The listing builds one solid part. Answer for the finished solid, in the listing's coordinates (mm). A direction names the side the tool comes from. Coordinates: 2 decimals unless noted, no trailing zeros. Loops run counter-clockwise (first coordinate to the right, second up) from the corner with the lowest first, then second, coordinate; pieces in that order, holes last. Notation, with made-up numbers: M 51.5,-19 L 93.5,-19 A23 ccw 93.5,4 Z; hole C -22,78.5 d7. An arc over 180 degrees is marked long. Return JSON: item names as keys, results as strings. Group by question number.
1. Section D-D (x = -5) is taken. Write down the section's boundary in (y, z), then the cut area to 3 significant figures.
2. Given P1, Ø1, axis at x = 4, z = 18, coming from the +Y side; P2, Ø3, axis at x = -1, z = 25, coming from the +Y side; P3, Ø7.5, axis at x = 4, z = -7, coming from the -Y side; P4, Ø3, axis at y = -2, z = -19.5, coming from the +X side, each flat-ended and moving along its own axis, determine where each tip first touches the part or whether it passes through.
3. The mould has two halves that part along Y. Classify faces 4 (the face through (0, 0, 0)), 5 (the face through (-2.4, -0.7, 0.1)), 6 (the face through (13.715, -6.505, -30.197)): pulls with the +Y half, pulls with the -Y half, needs draft (parallel to the pull), parting line crosses it, or undercut.
4. Section C-C (z = -25) is taken. Write down the section's boundary in (x, y).
5. Section B-B (x = -1) is taken. Write down the section's boundary in (y, z).
6. Straight lines are drawn through the part: L1, parallel to Z at x = -1, y = -0.9; L2, parallel to Y at x = 12.5, z = -30.5; L3, parallel to Z at x = -5, y = -0.95. For each, find the intervals that lie inside material, in ascending order. Write a range as from..to.
7. Which of the six approach directions +Z, -Z, +X, -X, +Y, -Y give full straight-line access (tool end or side, diameter ignored) to faces 1 (the face through (9.58, -2.38, 30.3)), 2 (the face through (12, -1, 26.5)), 3 (the face through (-0.662, -0.74, 27.578))?
8. Section A-A (y = -4.15) is taken. Write down the section's boundary in (x, z), then the cut area to 3 significant figures.
```python
from build123d import *

# Parameters (mm, degrees)
TABAN_FLAN_1_DEPTH    = 34
IZIM9_W               = 9.15
IZIM9_H               = 53
KES_EKSTR_ZYON1_DEPTH = 39.757096124
IZIM11_R              = 2.6
KES_EKSTR_ZYON2_DEPTH = 10
RADYUS1_R             = 2.5


# Sheet-metal steps are written as plain solids
with BuildPart() as part:
    # Çizim1 → Taban-Flanş1 (new, symmetric)
    with BuildSketch(Plane.XY):
        with BuildLine():
            Line((-12.5, 0), (12.5, 0))
            ThreePointArc((12.5, 0), (14.537154879, -7.765591238), (8.95035213, -2))
            Line((8.95035213, -2), (10.233357384, -2.777108434))
            ThreePointArc((10.233357384, -2.777108434), (13.800833838, -6.458751031), (12.5, -1.5))
            Line((12.5, -1.5), (-12.5, -1.5))
            Line((-12.5, -1.5), (-12.5, 0))
        make_face()
    extrude(amount=TABAN_FLAN_1_DEPTH, both=True)

    # Çizim9 → Kes-Ekstrüzyon1 (cut, through all)
    with BuildSketch(Plane(origin=(0, 0, 0), x_dir=(1, 0, 0), z_dir=(0, 1, 0))):
        with Locations((12.075, 0)):
            Rectangle(IZIM9_W, IZIM9_H)
    extrude(amount=-KES_EKSTR_ZYON1_DEPTH, mode=Mode.SUBTRACT)

    # Çizim11 → Kes-Ekstrüzyon2 (cut)
    with BuildSketch(Plane(origin=(0, 0, 0), x_dir=(1, 0, 0), z_dir=(0, 1, 0))):
        with Locations(Location((-1, 25, 0), (0, 0, 180))):
            Circle(IZIM11_R)
        with Locations(Location((-1, -25, 0), (0, 0, 180))):
            Circle(IZIM11_R)
        with Locations(Location((-5, 0, 0), (0, 0, 180))):
            Circle(IZIM11_R)
    extrude(amount=-KES_EKSTR_ZYON2_DEPTH, mode=Mode.SUBTRACT)

    # Radyus1
    radyus1_edges = [part.edges().sort_by_distance(p)[0] for p in [
        (-12.5, -0.75, 34),
        (-12.5, -0.75, -34),
    ]]
    fillet(radyus1_edges, radius=RADYUS1_R)


solid = part.part
```
Worked out:
{
 "1": {"outline": "M -1.5,-34 L 0,-34 L 0,-2.6 L -1.5,-2.6 Z; M -1.5,2.6 L 0,2.6 L 0,34 L -1.5,34 Z", "area": "94.2 mm^2"},
 "2": {"P1": "y = 0", "P2": "through", "P3": "y = -1.5", "P4": "x = 7.5"},
 "3": {"face 4": "pulls with the +Y half", "face 5": "needs draft", "face 6": "undercut"},
 "4": {"outline": "M -12.5,-1.5 L -3.6,-1.5 L -3.6,0 L -12.5,0 Z; M 1.6,-1.5 L 7.5,-1.5 L 7.5,0 L 1.6,0 Z"},
 "5": {"outline": "M -1.5,-34 L 0,-34 L 0,-27.6 L -1.5,-27.6 Z; M -1.5,-22.4 L 0,-22.4 L 0,22.4 L -1.5,22.4 Z; M -1.5,27.6 L 0,27.6 L 0,34 L -1.5,34 Z"},
 "6": {"L1": "-34..-27.6, -22.4..22.4, 27.6..34", "L2": "-8.3..-6.8, -1.5..0", "L3": "-34..-2.6, 2.6..34"},
 "7": {"face 1": "+Z, -Z", "face 2": "+X, +Y, -Y", "face 3": "+Y, -Y"},
 "8": {"outline": "M 8.35,-34 L 9.85,-34 L 9.85,-26.5 L 8.35,-26.5 Z; M 8.35,26.5 L 9.85,26.5 L 9.85,34 L 8.35,34 Z; M 15.15,-34 L 16.65,-34 L 16.65,-26.5 L 15.15,-26.5 Z; M 15.15,26.5 L 16.65,26.5 L 16.65,34 L 15.15,34 Z", "area": "45.0 mm^2"}
}
